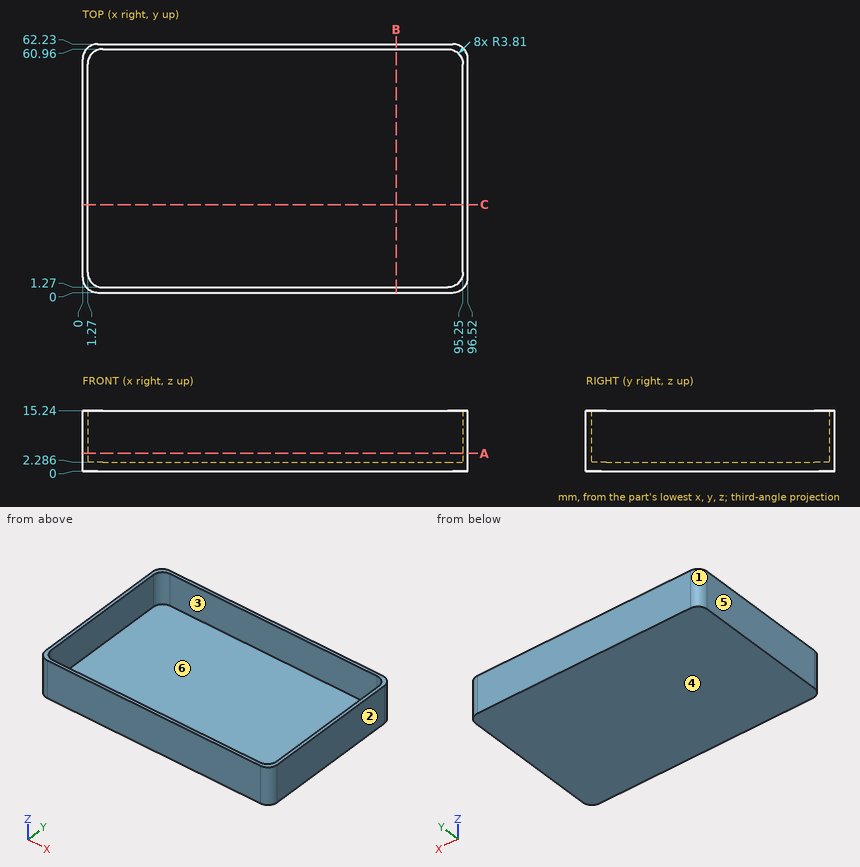
The figure shows three views and two pictorial views of one solid part (mm, origin at its lowest corner). Answer the questions. A direction names the side the tool comes from. Round coordinates to 2 decimals unless told otherwise and drop trailing zeros. Write each loop counter-clockwise with the first axis right and the second up, starting at its lowest first coordinate (ties: lowest second). Pieces come first, ordered by that corner, then holes. Notation, with made-up numbers: (4, -38) - (23, -38) arc R21 cw to (23, -18) - close; hole circle Ø3 at (46.25, -32). An arc over 180 degrees is marked (long way). Use one line per item in the form item = value. Start each with the question number.
Item 1: A tool of negligible diameter and unlimited length cuts with its end or side. For the marked faces 5 and 6, from which of +Z, -Z, +X, -X, +Y, -Y can it reach the whole face along a straight path? Write none if from no direction.
Item 2: Determine the mould class of the marked faces 1, 2, 3 and 4 for opening direction X: +X half, -X half, draft (parallel to the pull), parting line (faces both ways), or undercut.
Item 3: Flat-ended cylindrical pins translate along their axes: pin 1 Ø1 at (y, z) = (36, 8.5) entering from -X; pin 2 Ø8 at (x, y) = (40.5, 50) entering from +Z. Find the tip coordinate at first contact, or state that the pin passes through.
Item 4: A cutting plane is placed at C-C (y = 22). Write down the section's boundary in (x, z), plus the area to 3 significant figures.
Item 5: A cutting plane is placed at B-B (x = 78.5). Write down the section's boundary in (y, z).
Item 6: Find the intervals of material crossed by line 1 (Y direction, x = 22, z = 2.75); line 2 (X direction, y = 52.5, z = 10.5); line 3 (Z direction, x = 90, y = 20), in increasing order. Write a range as [from, to].
Item 7: A cutting plane is placed at A-A (z = 4.5). Write down the section's boundary in (x, y), plus the area to 3 significant figures.
The answers:
q1.face_5 = +Z, -Z, -X, +Y, -Y
q1.face_6 = +Z
q2.face_1 = -X half
q2.face_2 = +X half
q2.face_3 = undercut
q2.face_4 = draft
q3.pin_1 = 0
q3.pin_2 = 2.29
q4.outline = (0, 0) - (96.52, 0) - (96.52, 15.24) - (95.25, 15.24) - (95.25, 2.29) - (1.27, 2.29) - (1.27, 15.24) - (0, 15.24) - close
q4.area = 254 mm^2
q5.outline = (0, 0) - (62.23, 0) - (62.23, 15.24) - (60.96, 15.24) - (60.96, 2.29) - (1.27, 2.29) - (1.27, 15.24) - (0, 15.24) - close
q6.line_1 = [0, 1.27], [60.96, 62.23]
q6.line_2 = [0, 1.27], [95.25, 96.52]
q6.line_3 = [0, 2.29]
q7.outline = (0, 3.81) arc R3.81 ccw to (3.81, 0) - (92.71, 0) arc R3.81 ccw to (96.52, 3.81) - (96.52, 58.42) arc R3.81 ccw to (92.71, 62.23) - (3.81, 62.23) arc R3.81 ccw to (0, 58.42) - close; hole (1.27, 5.08) arc R3.81 ccw to (5.08, 1.27) - (91.44, 1.27) arc R3.81 ccw to (95.25, 5.08) - (95.25, 57.15) arc R3.81 ccw to (91.44, 60.96) - (5.08, 60.96) arc R3.81 ccw to (1.27, 57.15) - close
q7.area = 397 mm^2
